Can you work these out from the drawing? Everything is in mm from the part's minimum corner. Give positions to 0.01 mm unless a question says otherwise; leave off trailing zeros. Write each loop counter-clockwise with the first axis right and the second up, starting at its lowest first coordinate (ties: lowest second). Pieces come first, ordered by that corner, then holes. Notation, with made-up numbers: (9.25, 63.25) - (24.25, 63.25) arc R19 ccw to (24.25, 95.25) - close; hole circle Ø2 at (-37.75, 11). An arc over 180 degrees is marked (long way). Return JSON: item names as keys, results as strings. Group by question number.
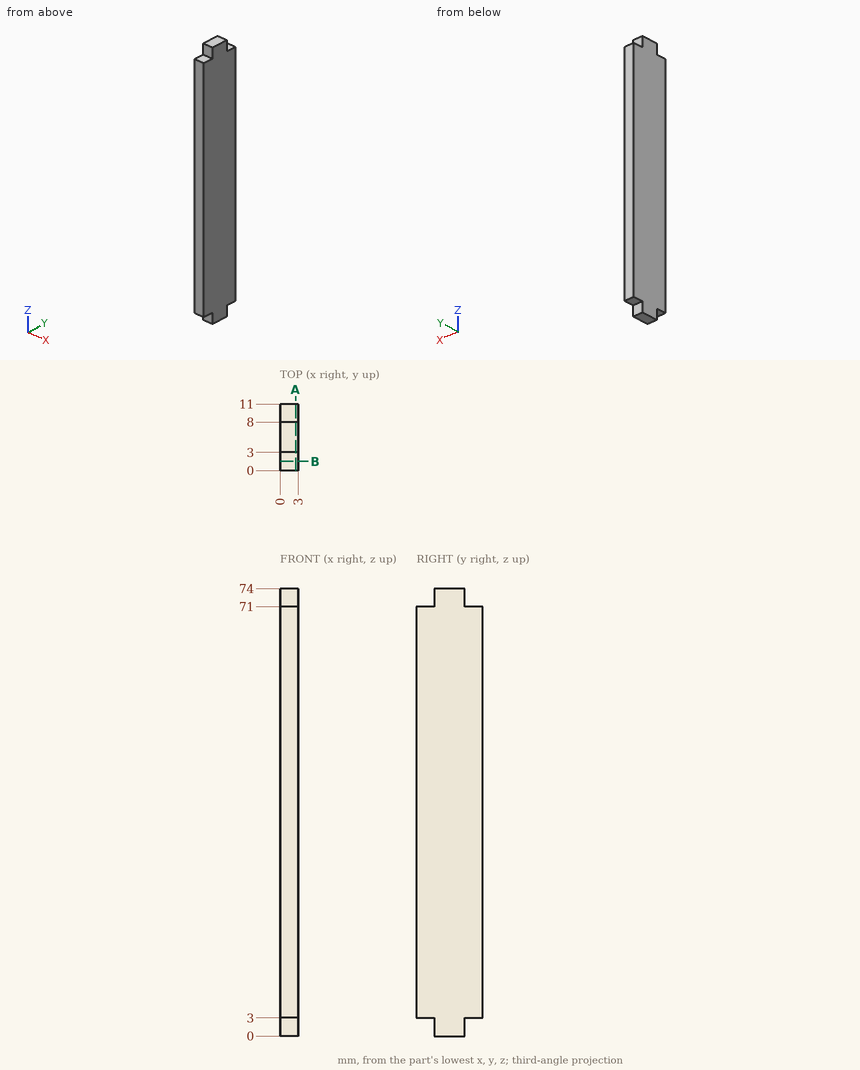
1) Imagine slicing it at A-A, the plane x = 2.55. Write out the boundary of the cut face in (y, z), and give its area (3 significant figures).
2) Will these pins go through, and if not, where does the flat tip stop? pin 1 Ø0.9 at (x, y) = (2, 9) entering from -Z; pin 2 Ø1.5 at (x, z) = (2, 73) entering from +Y; pin 3 Ø0.9 at (x, y) = (1.5, 2) entering from +Z.
3) Imagine slicing it at B-B, the plane y = 1.5. Write out the boundary of the cut face in (x, z).
4) I need wall thicknesses on line 1 along Z through (x, y) = (1.3, 1). Which ranges of the line are inside material? Lowest first, please.
Resolved:
{
 "1": {"outline": "(0, 3) - (3, 3) - (3, 0) - (8, 0) - (8, 3) - (11, 3) - (11, 71) - (8, 71) - (8, 74) - (3, 74) - (3, 71) - (0, 71) - close", "area": "778 mm^2"},
 "2": {"pin 1": "z = 3", "pin 2": "y = 8", "pin 3": "z = 71"},
 "3": {"outline": "(0, 3) - (3, 3) - (3, 71) - (0, 71) - close"},
 "4": {"line 1": "3 to 71"}
}
